Geometry check sheet. Reference: the model listing, model coordinates, mm. A direction names the side the tool comes from. Coordinates: 2 decimals unless noted, no trailing zeros. Write each loop counter-clockwise with the first axis right and the second up, starting at its lowest first coordinate (ties: lowest second). Pieces come first, ordered by that corner, then holes. Notation, with made-up numbers: (49, 8) -> (60, 8) arc R31 ccw to (60, 41) -> close; hole circle Ø9 at (66.25, 38). An arc over 180 degrees is marked (long way). Use a Markdown table: item, result.
```python
from build123d import *

# Parameters (mm, degrees)
EXTRUDE1_DEPTH     = 50.8
SKETCH2_R          = 3.175
CUT_EXTRUDE1_DEPTH = 88.988181024
SKETCH3_R          = 6.35
CUT_EXTRUDE2_DEPTH = 88.988181024


with BuildPart() as part:
    # Sketch1 → Extrude1 (new body)
    with BuildSketch(Plane.XY):
        Polygon((0, 0), (0, 50.8), (12.7, 50.8), (12.7, 12.7), (38.1, 12.7), (38.1, 50.8), (50.8, 50.8), (50.8, 0), align=None)
    extrude(amount=EXTRUDE1_DEPTH)

    # Sketch2 → Cut-Extrude1 (cut, through all)
    with BuildSketch(Plane.XZ):
        with Locations((25.4, 41.275)):
            Circle(SKETCH2_R)
        with Locations((25.4, 9.525)):
            Circle(SKETCH2_R)
    extrude(amount=-CUT_EXTRUDE1_DEPTH, mode=Mode.SUBTRACT)

    # Sketch3 → Cut-Extrude2 (cut, through all)
    with BuildSketch(Plane(origin=(50.8, 0, 0), x_dir=(0, 0, -1), z_dir=(1, 0, 0))):
        with Locations(Location((-25.4, 25.4, 0), (0, 0, 90))):
            Circle(SKETCH3_R)
    extrude(amount=-CUT_EXTRUDE2_DEPTH, mode=Mode.SUBTRACT)


solid = part.part
```
Item 1: Thickness scan on L1, parallel to Z at x = 25.4, y = 5.25; L2, parallel to X at y = 46, z = 17; L3, parallel to Z at x = 12, y = 25. Record the ranges inside material, lowest first. Write a range as [from, to].
Answer block:
| item | result |
|---|---|
| L1 | z = [0, 6.35], [12.7, 38.1], [44.45, 50.8] |
| L2 | x = [0, 12.7], [38.1, 50.8] |
| L3 | z = [0, 19.06], [31.74, 50.8] |
Item 2: Mould release check, pull along X, two halves, no side actions. Record for faces 3 (the flat face through (6, 50.8, 25)), 4 (the flat face through (0, 31, 31)), 5 (the cylindrical face through (28.43, 6.26, 42.23)), 6 (the flat face through (38.1, 36, 25)): +X half, -X half, draft (parallel to the pull), parting line (faces both ways), or undercut.
Answer block:
| item | result |
|---|---|
| face 3 | draft |
| face 4 | -X half |
| face 5 | undercut |
| face 6 | undercut |
Item 3: Depth check by flat-ended pin: P1, Ø7.5, axis at x = 25.4, z = 9.525, coming from the +Y side; P2, Ø4, axis at y = 18.5, z = 9.5, coming from the -X side; P3, Ø10, axis at y = 25.4, z = 25.4, coming from the -X side. Enter the tip coordinate at first touch or a pass-through.
Answer block:
| item | result |
|---|---|
| P1 | stops at y = 12.7 |
| P2 | stops at x = 0 |
| P3 | passes through |
Item 4: Tool access check on faces 1 (the flat face through (26, 0, 25)), 2 (the flat face through (12.7, 32, 25)). Record the directions out of +Z, -Z, +X, -X, +Y, -Y that give a thin tool (end or side, any length) a straight path to the whole face; none if there is none.
Answer block:
| item | result |
|---|---|
| face 1 | +Z, -Z, +X, -X, -Y |
| face 2 | +Z, -Z, +Y |
Item 5: Section check B-B on z = 25.4. Record the boundary of the cut face in (x, y), then the cut area to 3 significant figures.
Answer block:
| item | result |
|---|---|
| outline | (0, 0) -> (50.8, 0) -> (50.8, 19.05) -> (38.1, 19.05) -> (38.1, 12.7) -> (12.7, 12.7) -> (12.7, 19.05) -> (0, 19.05) -> close; (0, 31.75) -> (12.7, 31.75) -> (12.7, 50.8) -> (0, 50.8) -> close; (38.1, 31.75) -> (50.8, 31.75) -> (50.8, 50.8) -> (38.1, 50.8) -> close |
| area | 1,290 mm^2 |
Item 6: Section check D-D on y = 47. Record the boundary of the cut face in (x, z).
Answer block:
| item | result |
|---|---|
| outline | (0, 0) -> (12.7, 0) -> (12.7, 50.8) -> (0, 50.8) -> close; (38.1, 0) -> (50.8, 0) -> (50.8, 50.8) -> (38.1, 50.8) -> close |
Item 7: Section check A-A on y = 25.4. Record the boundary of the cut face in (x, z), then the cut area to 3 significant figures.
Answer block:
| item | result |
|---|---|
| outline | (0, 0) -> (12.7, 0) -> (12.7, 19.05) -> (0, 19.05) -> close; (0, 31.75) -> (12.7, 31.75) -> (12.7, 50.8) -> (0, 50.8) -> close; (38.1, 0) -> (50.8, 0) -> (50.8, 19.05) -> (38.1, 19.05) -> close; (38.1, 31.75) -> (50.8, 31.75) -> (50.8, 50.8) -> (38.1, 50.8) -> close |
| area | 968 mm^2 |
Item 8: Section check C-C on x = 25.4. Record the boundary of the cut face in (y, z), then the cut area to 3 significant figures.
Answer block:
| item | result |
|---|---|
| outline | (0, 0) -> (12.7, 0) -> (12.7, 6.35) -> (0, 6.35) -> close; (0, 12.7) -> (12.7, 12.7) -> (12.7, 38.1) -> (0, 38.1) -> close; (0, 44.45) -> (12.7, 44.45) -> (12.7, 50.8) -> (0, 50.8) -> close |
| area | 484 mm^2 |
